Work out the finished part from the listing and answer in its coordinate system (mm). Face numbers are marked on the shaded views. A direction names the side the tool comes from. Give positions to 0.01 mm unless a question says otherwise; leave off trailing zeros. Order: outer loops, then holes, each group sorted by start corner. A loop starts at its lowest first (then second) coordinate and runs counter-clockwise, first axis right, second up. Notation, with made-up numbers: (61, 68.25) - (107, 68.25) arc R11 ccw to (107, 87.25) - close; hole circle Ø4 at (49.25, 57.5). An arc over 180 degrees is marked (long way). Put each result on its own line as item: value.
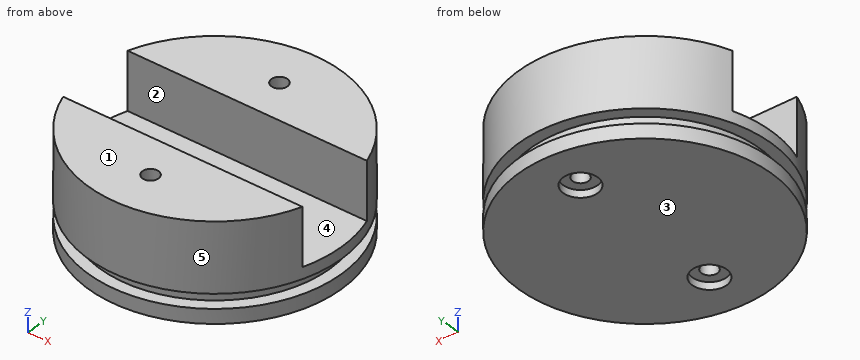
```python
from build123d import *

# Parameters (mm, degrees)
SKETCH1_R           = 22
BOSS_EXTRUDE1_DEPTH = 2.5
SKETCH2_R           = 20
BOSS_EXTRUDE2_DEPTH = 5
BOSS_EXTRUDE3_START = 5
SKETCH1_2_R         = 22
BOSS_EXTRUDE3_DEPTH = 12
CUT_EXTRUDE1_START  = 17
SKETCH3_W           = 56.338981098
SKETCH3_H           = 14
CUT_EXTRUDE1_DEPTH  = 10
SKETCH4_R           = 1.4
CUT_EXTRUDE2_DEPTH  = 18
SKETCH5_R           = 3
CUT_EXTRUDE3_DEPTH  = 1.3


with BuildPart() as part:
    # Sketch1 → Boss-Extrude1 (new body)
    with BuildSketch(Plane.XY):
        Circle(SKETCH1_R)
    extrude(amount=BOSS_EXTRUDE1_DEPTH)

    # Sketch2 → Boss-Extrude2 (add)
    with BuildSketch(Plane.XY):
        Circle(SKETCH2_R)
    extrude(amount=BOSS_EXTRUDE2_DEPTH)

    # Sketch1<2> → Boss-Extrude3 (add)
    with BuildSketch(Plane.XY.offset(BOSS_EXTRUDE3_START)):
        Circle(SKETCH1_2_R)
    extrude(amount=BOSS_EXTRUDE3_DEPTH)

    # Sketch3 → Cut-Extrude1 (cut)
    with BuildSketch(Plane.XY.offset(CUT_EXTRUDE1_START)):
        with Locations((-1.268364496, 0)):
            Rectangle(SKETCH3_W, SKETCH3_H)
    extrude(amount=-CUT_EXTRUDE1_DEPTH, mode=Mode.SUBTRACT)

    # Sketch4 → Cut-Extrude2 (cut, through all)
    with BuildSketch(Plane.XY):
        with Locations((0, 14)):
            Circle(SKETCH4_R)
        with Locations((0, -14)):
            Circle(SKETCH4_R)
    extrude(amount=CUT_EXTRUDE2_DEPTH, mode=Mode.SUBTRACT)

    # Sketch5 → Cut-Extrude3 (cut)
    with BuildSketch(Plane.XY):
        with Locations((0, 14)):
            Circle(SKETCH5_R)
        with Locations((0, -14)):
            Circle(SKETCH5_R)
    extrude(amount=CUT_EXTRUDE3_DEPTH, mode=Mode.SUBTRACT)


solid = part.part
```
(1) Section A-A, the plane x = 0 is taken. Count the separate pieces of the cut face and the enclosed holes in it, then the cut area to 3 significant figures.
Geometry check:
separate pieces: 3
enclosed holes: 0
area: 494 mm²
(2) Section D-D, the plane y = -14 is taken. Write down the section's boundary in (x, z), then the cut area to 3 significant figures.
Geometry check:
outline: (-16.97, 0) - (-3, 0) - (-3, 1.3) - (-1.4, 1.3) - (-1.4, 17) - (-16.97, 17) - (-16.97, 5) - (-14.28, 5) - (-14.28, 2.5) - (-16.97, 2.5) - close; (1.4, 1.3) - (3, 1.3) - (3, 0) - (16.97, 0) - (16.97, 2.5) - (14.28, 2.5) - (14.28, 5) - (16.97, 5) - (16.97, 17) - (1.4, 17) - close
area: 512 mm²
(3) Determine the mould class of the marked faces 3, 4 and 5 for opening direction Y: pulls with the +Y half, pulls with the -Y half, needs draft (parallel to the pull), parting line crosses it, or undercut.
Geometry check:
face 3: needs draft
face 4: undercut
face 5: parting line crosses it
(4) Straight lines are drawn through the part: line 1 (Y direction, x = 0, z = 0.9); line 2 (Y direction, x = 0, z = 13.75); line 3 (Y direction, x = 7, z = 12.25). For each, find the intervals that lie inside material, in ascending order.
Geometry check:
line 1: y = -22 to -17, -11 to 11, 17 to 22
line 2: y = -22 to -15.4, -12.6 to -7, 7 to 12.6, 15.4 to 22
line 3: y = -20.86 to -7, 7 to 20.86
(5) Given pin 1 (6 mm diameter, centred on x = -10, z = 13, fed in from +Y); pin 2 (1 mm diameter, centred on x = -9, z = 11.5, fed in from -Y); pin 3 (2 mm diameter, centred on x = 10, z = 5.5, fed in from -Y), each flat-ended and moving along its own axis, determine where each tip first touches the part or whether it passes through.
Geometry check:
pin 1: stops at y = 20.86
pin 2: stops at y = -20.29
pin 3: stops at y = -20.07
(6) Section B-B, the plane z = 12.75 is taken. Write down the section's boundary in (x, y), then the cut area to 3 significant figures.
Geometry check:
outline: (-20.86, -7) arc R22 ccw to (20.86, -7) - close; (-20.86, 7) - (20.86, 7) arc R22 ccw to start; hole circle Ø2.8 at (0, -14); hole circle Ø2.8 at (0, 14)
area: 903 mm²
(7) A tool of negligible diameter and unlimited length cuts with its end or side. For the marked faces 1 and 2, from which of +Z, -Z, +X, -X, +Y, -Y can it reach the whole face along a straight path? Write none if from no direction.
Geometry check:
face 1: +Z, +X, -X, +Y, -Y
face 2: +Z, +X, -X
(8) Section C-C, the plane y = 0 is taken. Write down the section's boundary in (x, z), then the cut area to 3 significant figures.
Geometry check:
outline: (-22, 0) - (22, 0) - (22, 2.5) - (20, 2.5) - (20, 5) - (22, 5) - (22, 7) - (-22, 7) - (-22, 5) - (-20, 5) - (-20, 2.5) - (-22, 2.5) - close
area: 298 mm²
